Input: part model. Units: mm. Frame: model coordinates. Face numbers are marked on the shaded views. A direction names the side the tool comes from. Round coordinates to 2 decimals unless told otherwise and drop trailing zeros. Write each loop counter-clockwise with the first axis right and the second up, starting at its lowest first coordinate (ties: lowest second). Pieces come first, ordered by that corner, then holes. Notation, with made-up numbers: (-11.75, 21.25) -> (34.25, 21.25) arc R10 cw to (34.25, 33.25) -> close; hole circle Ø10 at (-40, 47). An arc over 180 degrees is marked (long way). Write item = value, one per line. Start each with the question number.
Autodesk Fusion 360 part; units mm, degrees
sketch "Sketch1" plane through (0, 0, 0) normal (0, 1, 0) x (1, 0, 0)
  line L0 (0, 0) -> (20, 0)
  line L1 (0, 20) -> (0, 0)
  line L2 (20, 0) -> (40, 0)
  line L3 (40, 0) -> (60, 0)
  line L4 (60, 0) -> (80, 0)
  line L5 (80, 20) -> (60, 20)
  line L6 (80, 0) -> (80, 20)
  line L7 (0, 40) -> (0, 20)
  line L8 (0, 60) -> (0, 40)
  line L9 (20, 80) -> (0, 80)
  line L10 (20, 80) -> (20, 60)
  line L11 (0, 80) -> (0, 60)
  line L12 (40, 60) -> (20, 60)
  line L13 (40, 40) -> (40, 60)
  line L14 (60, 40) -> (40, 40)
  line L15 (60, 40) -> (60, 20)
  point P0 (20, 0)
  point P1 (40, 0)
  point P2 (60, 0)
  dimension "d1" = 20
  dimension "d2" = 20
extrude "Extrude1" add sketch "Sketch1" along normal blind 20
sketch "Sketch2" plane through (0, 20, 0) normal (0, 1, 0) x (-1, 0, 0)
  line L0 (-40, -40) -> (-40, -60)
  line L1 (-40, -60) -> (-20, -60)
  line L2 (-20, -60) -> (-20, -80)
  line L3 (-20, -80) -> (0, -80)
  line L4 (0, -80) -> (0, 0)
  line L5 (0, 0) -> (-80, 0)
  line L6 (-80, 0) -> (-80, -20)
  line L7 (-80, -20) -> (-60, -20)
  line L8 (-60, -20) -> (-60, -40)
  line L9 (-60, -40) -> (-40, -40)
  line L10 (0, 0) -> (-20, 0)
  line L11 (-20, -40) -> (-20, -60)
  line L12 (-20, -60) -> (0, -60)
  line L13 (0, -60) -> (0, 0)
  line L14 (-20, 0) -> (-40, 0)
  line L15 (-40, -40) -> (-20, -40)
  line L16 (-40, 0) -> (-60, 0)
  line L17 (-60, 0) -> (-60, -20)
  line L18 (-60, -20) -> (-40, -20)
  line L19 (-40, -20) -> (-40, -40)
  dimension "d21" = 20
  dimension "d22" = 60
  dimension "d23" = 20
  dimension "d24" = 40
  dimension "d25" = 20
  dimension "d26" = 20
extrude "Extrude2" add sketch "Sketch2" along normal blind 20 contours L4 L5 L10 L11 L12 L13 L14 L15 L16 L17 L18 L19
sketch "Sketch3" plane through (0, 40, 0) normal (0, 1, 0) x (-1, 0, 0)
  line L0 (-40, -20) -> (-40, -40)
  line L1 (-40, -40) -> (-20, -40)
  line L2 (-20, -40) -> (-20, -60)
  line L3 (-20, -60) -> (0, -60)
  line L4 (0, -60) -> (0, 0)
  line L5 (0, 0) -> (-60, 0)
  line L6 (-60, 0) -> (-60, -20)
  line L7 (-60, -20) -> (-40, -20)
  line L8 (0, 0) -> (-40, 0)
  line L9 (-40, 0) -> (-40, -20)
  line L10 (-40, -20) -> (-20, -20)
  line L11 (0, -20) -> (0, 0)
  line L12 (-20, -20) -> (-20, -40)
  line L13 (-20, -40) -> (0, -40)
  line L14 (0, -40) -> (0, -20)
  dimension "d29" = 40
  dimension "d30" = 20
  dimension "d31" = 20
  dimension "d32" = 20
extrude "Extrude3" add sketch "Sketch3" along normal blind 20 contours L4 L5 L8 L9 L10 L11 L12 L13 L14
sketch "Sketch4" plane through (0, 60, 0) normal (0, 1, 0) x (-1, 0, 0)
  line L0 (0, -40) -> (0, 0)
  line L1 (0, 0) -> (-40, 0)
  line L2 (-40, 0) -> (-40, -20)
  line L3 (-40, -20) -> (-20, -20)
  line L4 (-20, -20) -> (-20, -40)
  line L5 (-20, -40) -> (0, -40)
  line L6 (0, 0) -> (-20, 0)
  line L7 (-20, 0) -> (-20, -20)
  line L8 (-20, -20) -> (0, -20)
  line L9 (0, -20) -> (0, 0)
  dimension "d35" = 20
  dimension "d36" = 20
extrude "Extrude4" add sketch "Sketch4" along normal blind 20 contours L0 L1 L6 L7 L8 L9
shell "Shell1" thickness 4 removed faces 1 at (20, 0, -33.3333)
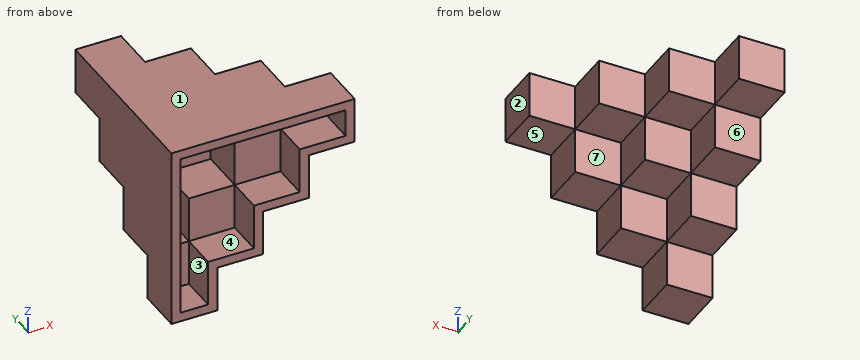
1. Mould query, pull axis Z, two halves, no side actions, for the marked faces 1, 2 and 3. Classes: pulls with the +Z half, pulls with the -Z half, needs draft (parallel to the pull), parting line crosses it, or undercut.
2. Section A-A (y = 54). Output: boundary loops of the cut face in (x, z), then the cut area to 3 significant figures.
3. Section C-C (z = -18.5). Output: boundary loops of the cut face in (x, y), then the cut area to 3 significant figures.
4. Line query: line 1 along X through (y, z) = (14, -48); line 2 along Z through (x, y) = (30.5, 41); line 3 along X through (y, z) = (47.5, -22). Output: solid intervals per line, ascending.
5. Reachability of the marked faces 4, 5, 6 and 7 from +Z, -Z, +X, -X, +Y, -Y: full face, straight path, thin tool, end or side. Return the list, or none.
6. Section D-D (y = 72). Output: boundary loops of the cut face in (x, z).
7. Section B-B (x = 62.5). Output: boundary loops of the cut face in (y, z), then the cut area to 3 significant figures.
8. Pin query (flat end, axial travel): P1, Ø6, axis at x = 13, y = 25, coming from the -Z side; P2, Ø6, axis at y = 50, z = -7, coming from the +X side; P3, Ø6, axis at x = 28, z = -26, coming from the -Y side. Return the tip coordinate at first contact, or that it passes through.
Check sheet entries:
q1.face_1 = pulls with the +Z half
q1.face_2 = needs draft
q1.face_3 = undercut
q2.outline = (0, -40) -> (20, -40) -> (20, -20) -> (40, -20) -> (40, 0) -> (0, 0) -> close; hole (4, -36) -> (16, -36) -> (16, -16) -> (36, -16) -> (36, -4) -> (4, -4) -> close
q2.area = 576 mm2
q3.outline = (0, 0) -> (4, 0) -> (4, 56) -> (16, 56) -> (16, 36) -> (36, 36) -> (36, 16) -> (56, 16) -> (56, 0) -> (80, 0) -> (80, 20) -> (60, 20) -> (60, 40) -> (40, 40) -> (40, 60) -> (20, 60) -> (20, 80) -> (0, 80) -> close
q3.area = 2,290 mm2
q4.line_1 = 0 to 4, 36 to 40
q4.line_2 = -20 to -16, -4 to 0
q4.line_3 = 0 to 4, 16 to 20
q5.face_4 = -Y
q5.face_5 = -Z, +X, +Y, -Y
q5.face_6 = -Z, +X, -X, +Y
q5.face_7 = -Z, +X, +Y
q6.outline = (0, -20) -> (20, -20) -> (20, 0) -> (0, 0) -> close; hole (4, -16) -> (16, -16) -> (16, -4) -> (4, -4) -> close
q7.outline = (0, -20) -> (20, -20) -> (20, 0) -> (0, 0) -> (0, -4) -> (16, -4) -> (16, -16) -> (0, -16) -> close
q7.area = 208 mm2
q8.P1 = -60
q8.P2 = 40
q8.P3 = 36
